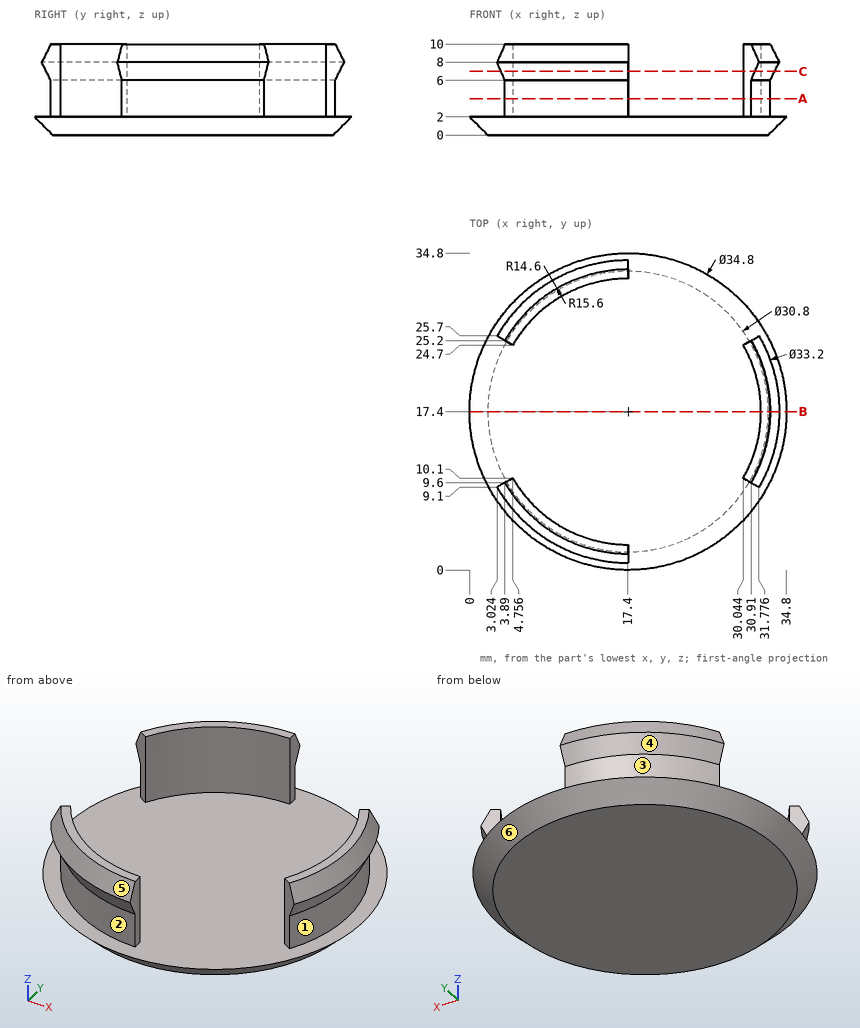
Could you check a few things on this drawing? It's one solid part, dimensions in mm from its lowest x, y, z. A direction names the side the tool comes from. Coordinates: 2 decimals unless noted, no trailing zeros. Loops run counter-clockwise (first coordinate to the right, second up) from the corner with the lowest first, then second, coordinate; pieces in that order, holes last. Notation, with made-up numbers: (83, 65.5) - (110, 65.5) arc R18 cw to (110, 91.5) - close; hole circle Ø3 at (49, 3.5). An arc over 180 degrees is marked (long way). Answer as a JSON object with one key per item and string values. Group by question number.
Item 1: For pin 1 (0.6 mm diameter, centred on y = 2, z = 7, fed in from +X); pin 2 (12 mm diameter, centred on x = 13.5, y = 18.5, fed in from +Z); pin 3 (1.5 mm diameter, centred on y = 19.5, z = 3.5, fed in from -X), each with a flat end and sliding along its axis, tell me the tip position at first contact or that it passes through.
Item 2: If I drill on L1, parallel to Z at x = 12, y = 28.5; L2, parallel to Y at x = 5, z = 7.75; L3, parallel to Z at x = 4, y = 8.5, over which ranges is the centre line in solid material (lowest first)? Write a range as from..to.
Item 3: If we section it at B-B (y = 17.4): List the corners of the cut face in (x, z) for me.
Item 4: On a 3-axis mill with a long thin cutter (end or side, diameter ignored), from which of +Z, -Z, +X, -X, +Y, -Y can I reach the whole of each face in a straight line? I mean the marked faces 1, 2 and 3. Say none if no direction works.
Item 5: If we section it at A-A (z = 4): List the corners of the cut face in (x, y) for me.
Item 6: If we section it at C-C (z = 7): List the corners of the cut face in (x, y) for me.
Item 7: If we mould it in two halves opening along Z, with no side actions, what happens to the marked faces 4, 5 and 6? For each: released by +Z, released by -Z, zero draft, split by the parting line, or undercut.
Returned:
{
 "1": {"pin 1": "stops at x = 17.4", "pin 2": "stops at z = 2", "pin 3": "stops at x = 31.72"},
 "2": {"L1": "z = 0..2", "L2": "y = 6.55..9.69, 25.11..28.25", "L3": "z = 0.69..2, 6.97..9.03"},
 "3": {"outline": "(0, 2) - (2, 0) - (32.8, 0) - (34.8, 2) - (33, 2) - (33, 6) - (34, 8) - (33, 10) - (32, 10) - (32, 2) - close"},
 "4": {"face 1": "+X", "face 2": "-X, -Y", "face 3": "-X, +Y"},
 "5": {"outline": "(3.89, 9.6) arc R15.6 ccw to (17.4, 1.8) - (17.4, 2.8) arc R14.6 cw to (4.76, 10.1) - close; (3.89, 25.2) - (4.76, 24.7) arc R14.6 cw to (17.4, 32) - (17.4, 33) arc R15.6 ccw to start; (30.04, 10.1) - (30.91, 9.6) arc R15.6 ccw to (30.91, 25.2) - (30.04, 24.7) arc R14.6 cw to start"},
 "6": {"outline": "(3.46, 9.35) arc R16.1 ccw to (17.4, 1.3) - (17.4, 2.8) arc R14.6 cw to (4.76, 10.1) - close; (3.46, 25.45) - (4.76, 24.7) arc R14.6 cw to (17.4, 32) - (17.4, 33.5) arc R16.1 ccw to start; (30.04, 10.1) - (31.34, 9.35) arc R16.1 ccw to (31.34, 25.45) - (30.04, 24.7) arc R14.6 cw to start"},
 "7": {"face 4": "undercut", "face 5": "released by +Z", "face 6": "released by -Z"}
}
